Geometry: final body of the model. Coordinates: model frame, mm. Round coordinates to 2 decimals unless told otherwise and drop trailing zeros. Loops run counter-clockwise (first coordinate to the right, second up) from the corner with the lowest first, then second, coordinate; pieces in that order, holes last. Notation, with made-up numbers: M 78.25,20.25 L 117.25,20.25 A22 ccw 117.25,39.25 Z; hole C -40,68.5 d6. An arc over 180 degrees is marked long. Return JSON: item names as keys, results as strings.
from build123d import *

# Parameters (mm, degrees)
SKETCH_1_W          = 330
SKETCH_1_H          = 390
EXTRUDE_1_DEPTH     = 4
SKETCH_3_W          = 110
SKETCH_3_H          = 110
CUT_EXTRUDE_1_DEPTH = 4
SKETCH_5_R          = 1.25
CUT_EXTRUDE_2_DEPTH = 4
SKETCH_7_R          = 2
CUT_EXTRUDE_3_DEPTH = 4
SKETCH_8_R          = 1.6
CUT_EXTRUDE_4_DEPTH = 4
SKETCH_9_R          = 3
CUT_EXTRUDE_5_DEPTH = 4
SKETCH_11_R         = 3
CUT_EXTRUDE_6_DEPTH = 4
SKETCH_14_R         = 12.5
CUT_EXTRUDE_7_DEPTH = 4
FILLET_1_R          = 15
SKETCH_15_R         = 1.25
CUT_EXTRUDE_8_DEPTH = 4
CUT_EXTRUDE_9_DEPTH = 4


with BuildPart() as part:
    # 草图1 → 凸台-拉伸1 (new body)
    with BuildSketch(Plane.XY):
        Rectangle(SKETCH_1_W, SKETCH_1_H)
    extrude(amount=EXTRUDE_1_DEPTH)

    # 草图3 → 切除-拉伸1 (cut)
    with BuildSketch(Plane.XY.offset(4)):
        with Locations((165, 125)):
            Rectangle(SKETCH_3_W, SKETCH_3_H)
        with Locations((165, -125)):
            Rectangle(SKETCH_3_W, SKETCH_3_H)
        with Locations((-165, -125)):
            Rectangle(SKETCH_3_W, SKETCH_3_H)
        with Locations((-165, 125)):
            Rectangle(SKETCH_3_W, SKETCH_3_H)
    extrude(amount=-CUT_EXTRUDE_1_DEPTH, mode=Mode.SUBTRACT)

    # 草图5 → 切除-拉伸2 (cut)
    with BuildSketch(Plane.XY.offset(4)):
        with Locations((24.5, -163)):
            Circle(SKETCH_5_R)
        with Locations((24.5, -105)):
            Circle(SKETCH_5_R)
        with Locations(Location((-24.5, -105, 0), (0, 0, 180))):
            Circle(SKETCH_5_R)
        with Locations(Location((-24.5, -163, 0), (0, 0, 180))):
            Circle(SKETCH_5_R)
    extrude(amount=-CUT_EXTRUDE_2_DEPTH, mode=Mode.SUBTRACT)

    # 草图7 → 切除-拉伸3 (cut)
    with BuildSketch(Plane.XY.offset(4)):
        with Locations((49.493881146, 0)):
            Circle(SKETCH_7_R)
        with Locations((-49.501067959, 0.007186813)):
            Circle(SKETCH_7_R)
        with Locations((0, 49.501067959)):
            Circle(SKETCH_7_R)
        with Locations((-0.007186813, -49.493881146)):
            Circle(SKETCH_7_R)
    extrude(amount=-CUT_EXTRUDE_3_DEPTH, mode=Mode.SUBTRACT)

    # 草图8 → 切除-拉伸4 (cut)
    with BuildSketch(Plane.XY.offset(4)):
        with Locations((24.75, 121.25952533)):
            Circle(SKETCH_8_R)
        with Locations((24.75, 147.25952533)):
            Circle(SKETCH_8_R)
        with Locations(Location((-24.75, 147.25952533, 0), (0, 0, 180))):
            Circle(SKETCH_8_R)
        with Locations(Location((-24.75, 121.25952533, 0), (0, 0, 180))):
            Circle(SKETCH_8_R)
    extrude(amount=-CUT_EXTRUDE_4_DEPTH, mode=Mode.SUBTRACT)

    # 草图9 → 切除-拉伸5 (cut)
    with BuildSketch(Plane.XY.offset(4)):
        with Locations((99, -140)):
            Circle(SKETCH_9_R)
        with Locations((75, -140)):
            Circle(SKETCH_9_R)
        with Locations(Location((99, -110, 0), (0, 0, 180))):
            Circle(SKETCH_9_R)
        with Locations(Location((75, -110, 0), (0, 0, 180))):
            Circle(SKETCH_9_R)
        with Locations((-99, -110)):
            Circle(SKETCH_9_R)
        with Locations((-75, -110)):
            Circle(SKETCH_9_R)
        with Locations(Location((-99, -140, 0), (0, 0, 180))):
            Circle(SKETCH_9_R)
        with Locations(Location((-75, -140, 0), (0, 0, 180))):
            Circle(SKETCH_9_R)
    extrude(amount=-CUT_EXTRUDE_5_DEPTH, mode=Mode.SUBTRACT)

    # 草图11 → 切除-拉伸6 (cut)
    with BuildSketch(Plane.XY.offset(4)):
        with Locations((99, 140)):
            Circle(SKETCH_11_R)
        with Locations((99, 110)):
            Circle(SKETCH_11_R)
        with Locations((75, 110)):
            Circle(SKETCH_11_R)
        with Locations((75, 140)):
            Circle(SKETCH_11_R)
        with Locations(Location((-75, 110, 0), (0, 0, 180))):
            Circle(SKETCH_11_R)
        with Locations(Location((-99, 110, 0), (0, 0, 180))):
            Circle(SKETCH_11_R)
        with Locations(Location((-99, 140, 0), (0, 0, 180))):
            Circle(SKETCH_11_R)
        with Locations(Location((-75, 140, 0), (0, 0, 180))):
            Circle(SKETCH_11_R)
    extrude(amount=-CUT_EXTRUDE_6_DEPTH, mode=Mode.SUBTRACT)

    # 草图14 → 切除-拉伸7 (cut)
    with BuildSketch(Plane.XY.offset(4)):
        with Locations((45, 93.171201499)):
            Circle(SKETCH_14_R)
        with Locations((45, -75.052125949)):
            Circle(SKETCH_14_R)
        with Locations(Location((-45, -75.052125949, 0), (0, 0, 180))):
            Circle(SKETCH_14_R)
        with Locations(Location((-45, 93.171201499, 0), (0, 0, 180))):
            Circle(SKETCH_14_R)
    extrude(amount=-CUT_EXTRUDE_7_DEPTH, mode=Mode.SUBTRACT)

    # 圆角1
    fillet_1_edges = [part.edges().sort_by_distance(p)[0] for p in [
        (165, -195, 2),
        (-165, -195, 2),
        (165, 195, 2),
        (-165, 195, 2),
    ]]
    fillet(fillet_1_edges, radius=FILLET_1_R - 0.0001)  # a hair under: the kernel refuses the full size

    # 草图15 → 切除-拉伸8 (cut)
    with BuildSketch(Plane.XY.offset(4)):
        with Locations((154, 18.45)):
            Circle(SKETCH_15_R)
        with Locations((154, -18.342402047)):
            Circle(SKETCH_15_R)
    cut_extrude_8 = extrude(amount=-CUT_EXTRUDE_8_DEPTH, mode=Mode.SUBTRACT)

    # 草图16 → 切除-拉伸9 (cut)
    with BuildSketch(Plane.XY.offset(4)):
        Polygon((165, -12.5), (165, 12.5), (149, 12.5), (149, 22.5), (129, 22.5), (129, -22.5), (149, -22.5), (149, -12.5), align=None)
    cut_extrude_9 = extrude(amount=-CUT_EXTRUDE_9_DEPTH, mode=Mode.SUBTRACT)

    # 镜向1: 切除-拉伸8, 切除-拉伸9 across plane
    add(cut_extrude_8.mirror(Plane(origin=(0, 0, 0), x_dir=(0, 0, 1), z_dir=(1, 0, 0))), mode=Mode.SUBTRACT)
    add(cut_extrude_9.mirror(Plane(origin=(0, 0, 0), x_dir=(0, 0, 1), z_dir=(1, 0, 0))), mode=Mode.SUBTRACT)


solid = part.part
Q1. Section query A-A (y = 131.5). Output: boundary loops of the cut face in (x, z).
Determined:
{"outline": "M -110,0 L 110,0 L 110,4 L -110,4 Z"}
Q2. Pin query (flat end, axial travel): pin 1 (2 mm diameter, centred on x = -154, y = -18.34, fed in from +Z). Return the tip coordinate at first contact, or that it passes through.
Determined:
{"pin 1": "passes through"}
Q3. Material intervals for L1, parallel to Y at x = -99, z = 2.95; L2, parallel to Y at x = -24.5, z = 1.35; L3, parallel to Y at x = 45, z = 0.9, sorted ascending.
Determined:
{"L1": "y = -195 to -143, -137 to -113, -107 to 107, 113 to 137, 143 to 195", "L2": "y = -195 to -164.25, -161.75 to -106.25, -103.75 to 119.68, 122.84 to 145.68, 148.84 to 195", "L3": "y = -195 to -87.55, -62.55 to 80.67, 105.67 to 195"}
Q4. Section query B-B (z = 0.8). State how many separate pieces and enclosed holes the cut face has, plus the area to 3 significant figures.
Determined:
{"separate pieces": "1", "enclosed holes": "36", "area": "99,200 mm^2"}
Q5. Pull-direction query (Y, two-part tool) for faces 1 (the cylindrical face through (42.29, -87.255, 2.028)), 2 (the cylindrical face through (-160.72, -190.49, 2.03)), 3 (the cylindrical face through (160.49, 190.72, 2.03)), 4 (the cylindrical face through (-43.373, -87.446, 2.028)); classes: pulls with the +Y half, pulls with the -Y half, needs draft (parallel to the pull), parting line crosses it, or undercut.
Determined:
{"face 1": "undercut", "face 2": "pulls with the -Y half", "face 3": "pulls with the +Y half", "face 4": "undercut"}
